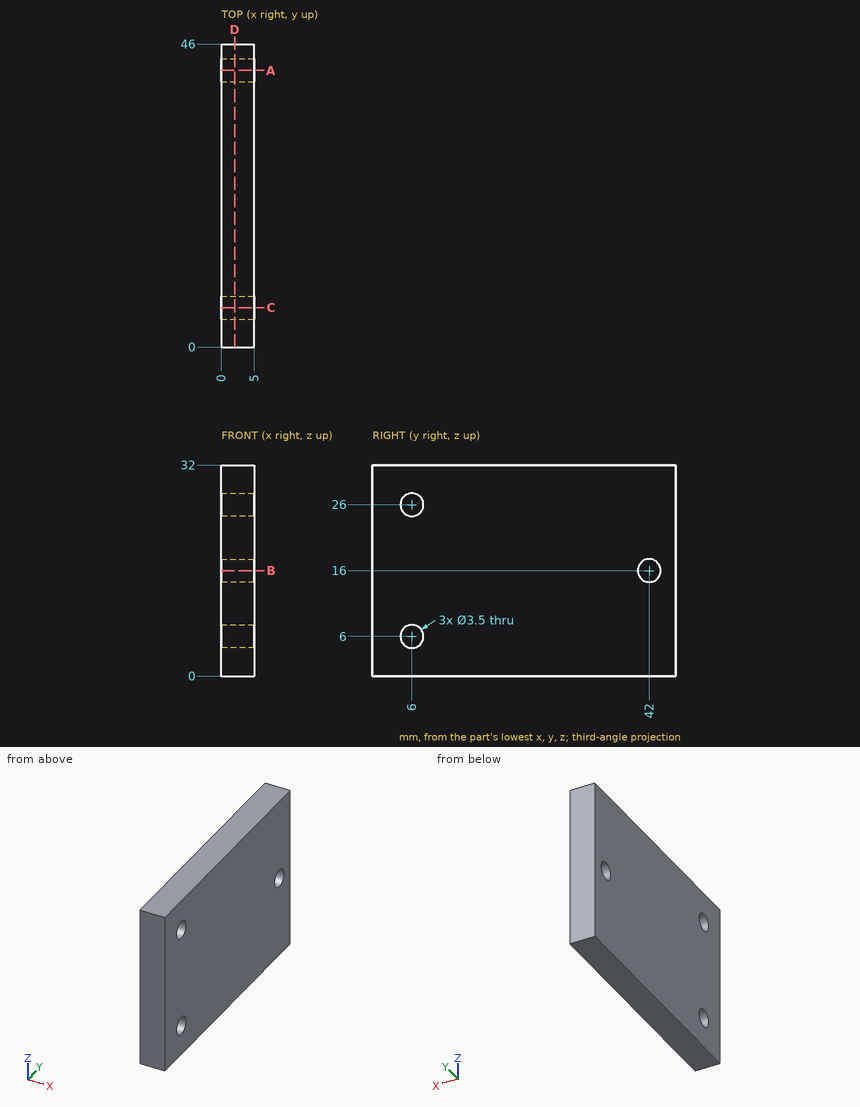
Part print with two shaded views. Sizes in mm from the minimum x, y, z corner. Coordinates: 2 decimals unless noted, no trailing zeros. Order: outer loops, then holes, each group sorted by start corner. A loop starts at its lowest first (then second) coordinate and runs counter-clockwise, first axis right, second up. Notation, with made-up numbers: M 18.25,56 L 61.25,56 A7 ccw 61.25,60 Z; hole C 65.25,71 d5. An arc over 180 degrees is marked long. One line per question, with ' | ' between items. Start each with the question number.
1. Cut at B-B (z = 16). Write the cut outline in (x, y).
2. Flat gauge pin, fed straight in: P1, Ø2, axis at y = 6, z = 26, coming from the -X side. Where does the tip first touch, or does it go through?
3. Wall check: line 1 along Y through (x, z) = (2.35, 6); line 2 along Y through (x, z) = (2.6, 16); line 3 along Z through (x, y) = (2.6, 43). Give the ranges that are in metal, low to high. Write a range as [from, to].
4. Cut at D-D (x = 2). Write the cut outline in (y, z).
5. Cut at A-A (y = 42). Write the cut outline in (x, z).
6. Cut at C-C (y = 6). Write the cut outline in (x, z).
The answers:
1) outline: M 0,0 L 5,0 L 5,40.25 L 0,40.25 Z; M 0,43.75 L 5,43.75 L 5,46 L 0,46 Z
2) P1: passes through
3) line 1: y = [0, 4.25], [7.75, 46] | line 2: y = [0, 40.25], [43.75, 46] | line 3: z = [0, 14.56], [17.44, 32]
4) outline: M 0,0 L 46,0 L 46,32 L 0,32 Z; hole C 6,6 d3.5; hole C 6,26 d3.5; hole C 42,16 d3.5
5) outline: M 0,0 L 5,0 L 5,14.25 L 0,14.25 Z; M 0,17.75 L 5,17.75 L 5,32 L 0,32 Z
6) outline: M 0,0 L 5,0 L 5,4.25 L 0,4.25 Z; M 0,7.75 L 5,7.75 L 5,24.25 L 0,24.25 Z; M 0,27.75 L 5,27.75 L 5,32 L 0,32 Z
